```python
from build123d import *

# Parameters (mm, degrees)
F1_DEPTH = 60


with BuildPart() as f1:
    # F0 (on Front) → F1 (new body)
    with BuildSketch(Plane.XZ):
        with BuildLine():
            ThreePointArc((-6.434941, 48.878232), (3.224374, 49.194445), (12.759779, 47.620143))
            Line((12.759779, 47.620143), (13.277417, 49.551995))
            ThreePointArc((13.277417, 49.551995), (5.162454, 51.039583), (-3.086029, 51.207094))
            ThreePointArc((-3.086029, 51.207094), (-4.087053, 51.136934), (-5.086513, 51.047207))
            Line((-5.086513, 51.047207), (-6.692654, 50.835755))
            Line((-6.692654, 50.835755), (-6.434941, 48.878232))
        make_face()
        with BuildLine():
            Line((-13.50154, 69.998845), (-10.266143, 50.262275))
            ThreePointArc((-10.266143, 50.262275), (-9.284233, 50.452879), (-8.298795, 50.624303))
            Line((-8.298795, 50.624303), (-11.527883, 70.322385))
            Line((-11.527883, 70.322385), (-13.50154, 69.998845))
        make_face()
        with BuildLine():
            ThreePointArc((-5.086513, 51.047207), (-4.087053, 51.136934), (-3.086029, 51.207094))
            Line((-3.086029, 51.207094), (-6.321426, 70.943664))
            Line((-6.321426, 70.943664), (-8.295083, 70.620124))
            Line((-8.295083, 70.620124), (-5.086513, 51.047207))
        make_face()
        with BuildLine():
            Line((-25.65, 44.427103), (-24.65, 42.695052))
            ThreePointArc((-24.65, 42.695052), (-15.846966, 46.683655), (-6.434941, 48.878232))
            Line((-6.434941, 48.878232), (-6.692654, 50.835755))
            Line((-6.692654, 50.835755), (-8.298795, 50.624303))
            ThreePointArc((-8.298795, 50.624303), (-9.284233, 50.452879), (-10.266143, 50.262275))
            ThreePointArc((-10.266143, 50.262275), (-18.193533, 47.96546), (-25.65, 44.427103))
        make_face()
    extrude(amount=F1_DEPTH)


solid = f1.part
```
Source: CAD feature listing. Evaluate the final solid. Frame: model axes, mm. A direction names the side the tool comes from. Coordinates: 2 decimals unless noted, no trailing zeros. Write each loop counter-clockwise with the first axis right and the second up, starting at its lowest first coordinate (ties: lowest second). Pieces come first, ordered by that corner, then holes. Notation, with made-up numbers: (31, 30.25) -> (45, 30.25) arc R25 cw to (45, 59.25) -> close; hole circle Ø2 at (-0.75, -24.75). An arc over 180 degrees is marked (long way). Return JSON: item names as keys, results as strings. Group by question number.
1) Section query D-D, the plane z = 45.75. Return loops of the section in (x, y).
2) Section query A-A, the plane z = 66.5. Return loops of the section in (x, y).
3) Ray query, line 1 along X through (y, z) = (-12.5, 59.5); line 2 along X through (y, z) = (-30.5, 57.75); line 3 along Z through (x, y) = (0, -31.5). Return the intervals inside material, ascending.
4) Section query C-C, the plane x = -2. Return loops of the section in (y, z).
5) Contact query for flat-ended pins moving along their axis: P1, Ø1.5, axis at x = 4.5, y = -43.5, coming from the -Z side; P2, Ø5, axis at x = -21, y = -41.5, coming from the -Z side; P3, Ø6, axis at y = -11.5, z = 62.5, coming from the +X side. Output: stop coordinate, or through.
6) Section query B-B, the plane y = -42. Return loops of the section in (x, z), plus the area to 3 significant figures.
7) Set-up query: faces 1 (the face through (-15.98, -29.58, 46.64)), 2 (the face through (-18.1, -29.6, 48)), 3 (the face through (-6.713, -29.58, 60.971)). Return all of +Z, -Z, +X, -X, +Y, -Y with unobstructed straight access to the full face (end or side cutting, diameter ignored); none if empty.
8) Mould query, pull axis X, two halves, no side actions, for faces 4 (the face through (13.015, -29.58, 48.573)), 5 (the face through (-9.2, -60, 54.8)), 6 (the face through (-11.906, -29.58, 60.269)), 7 (the face through (-9.89, -29.58, 60.34)). Classes: +X half, -X half, draft (parallel to the pull), parting line (faces both ways), or undercut.
From the geometry:
{
 "1": {"outline": "(-23.21, -60) -> (-18.37, -60) -> (-18.37, 0) -> (-23.21, 0) -> close"},
 "2": {"outline": "(-12.93, -60) -> (-10.9, -60) -> (-10.9, 0) -> (-12.93, 0) -> close; (-7.62, -60) -> (-5.59, -60) -> (-5.59, 0) -> (-7.62, 0) -> close"},
 "3": {"line 1": "-11.78 to -9.75, -6.47 to -4.45", "line 2": "-11.49 to -9.47, -6.19 to -4.16", "line 3": "49.3 to 51.3"},
 "4": {"outline": "(-60, 49.26) -> (0, 49.26) -> (0, 51.26) -> (-60, 51.26) -> close"},
 "5": {"P1": "z = 49.02", "P2": "z = 43.34", "P3": "x = -4.45"},
 "6": {"outline": "(-25.65, 44.43) -> (-24.65, 42.7) arc R49.3 cw to (-6.43, 48.88) arc R49.3 cw to (12.76, 47.62) -> (13.28, 49.55) arc R51.3 ccw to (-3.09, 51.21) -> (-6.32, 70.94) -> (-8.3, 70.62) -> (-5.09, 51.05) -> (-8.3, 50.62) -> (-11.53, 70.32) -> (-13.5, 70) -> (-10.27, 50.26) arc R51.3 ccw to start", "area": "159 mm²"},
 "7": {"face 1": "-Z, +Y, -Y", "face 2": "-X, +Y, -Y", "face 3": "+Y, -Y"},
 "8": {"face 4": "+X half", "face 5": "draft", "face 6": "-X half", "face 7": "undercut"}
}
